```python
from build123d import *

# Parameters (mm, degrees)
F0_W     = 145
F0_H     = 580
F1_DEPTH = 10
F2_W     = 125
F2_H     = 560
F3_DEPTH = 10
F4_R     = 1


with BuildPart() as f1:
    # F0 (on Top) → F1 (new body)
    with BuildSketch(Plane.XY):
        with Locations((-112.119565, 4.486432)):
            Rectangle(F0_W, F0_H)
    extrude(amount=F1_DEPTH)

    # F2 (on face) → F3 (join)
    with BuildSketch(Plane(origin=(0, 0, 0), x_dir=(1, 0, 0), z_dir=(0, 0, -1))):
        with Locations((-112.119565, -4.486432)):
            Rectangle(F2_W, F2_H)
    extrude(amount=F3_DEPTH)

    # F4
    f4_edges = [f1.edges().sort_by_distance(p)[0] for p in [
        (-49.619565, 4.486432, -10),
        (-112.119565, -275.513568, -10),
        (-174.619565, 4.486432, -10),
        (-112.119565, 284.486432, -10),
        (-184.619565, 4.486432, 0),
        (-49.619565, -275.513568, -5),
        (-174.619565, -275.513568, -5),
        (-112.119565, -275.513568, 0),
        (-49.619565, 284.486432, -5),
        (-49.619565, 4.486432, 0),
        (-39.619565, -285.513568, 5),
        (-39.619565, 294.486432, 5),
        (-39.619565, 4.486432, 0),
        (-39.619565, 4.486432, 10),
        (-184.619565, -285.513568, 5),
        (-112.119565, -285.513568, 0),
        (-112.119565, -285.513568, 10),
        (-184.619565, 294.486432, 5),
        (-184.619565, 4.486432, 10),
        (-112.119565, 294.486432, 0),
        (-112.119565, 294.486432, 10),
        (-174.619565, 284.486432, -5),
        (-112.119565, 284.486432, 0),
        (-174.619565, 4.486432, 0),
    ]]
    fillet(f4_edges, radius=F4_R)


solid = f1.part
```
Geometry check sheet. Reference: the model listing, model coordinates, mm. Coordinates: 2 decimals unless noted, no trailing zeros. Loops run counter-clockwise (first coordinate to the right, second up) from the corner with the lowest first, then second, coordinate; pieces in that order, holes last.
Item 1: Sectioned sample at C-C, the plane x = -141. Record the boundary of the cut face in (y, z).
Item 2: Sectioned sample at A-A, the plane y = -56.5. Record the boundary of the cut face in (x, z), then the cut area to 3 significant figures.
Item 3: Go/stop test with flat-tipped pins: pin 1 Ø2.5 at (x, z) = (-114, -4) entering from +Y; pin 2 Ø2 at (y, z) = (-95.5, -2) entering from -X; pin 3 Ø4 at (x, z) = (-140.5, -4.5) entering from -Y. Record where each tip stops, or that it passes through.
Item 4: Thickness scan on line 1 (X direction, y = -126, z = 9.25); line 2 (X direction, y = -84, z = -7); line 3 (Y direction, x = -56, z = -4). Record the ranges inside material, lowest first.
Item 5: Sectioned sample at B-B, the plane z = -6. Record the boundary of the cut face in (x, y), then the cut area to 3 significant figures.
Check result:
1. outline: (-285.51, 1) arc R1 ccw to (-284.51, 0) - (-276.51, 0) arc R1 cw to (-275.51, -1) - (-275.51, -9) arc R1 ccw to (-274.51, -10) - (283.49, -10) arc R1 ccw to (284.49, -9) - (284.49, -1) arc R1 cw to (285.49, 0) - (293.49, 0) arc R1 ccw to (294.49, 1) - (294.49, 9) arc R1 ccw to (293.49, 10) - (-284.51, 10) arc R1 ccw to (-285.51, 9) - close
2. outline: (-184.62, 1) arc R1 ccw to (-183.62, 0) - (-175.62, 0) arc R1 cw to (-174.62, -1) - (-174.62, -9) arc R1 ccw to (-173.62, -10) - (-50.62, -10) arc R1 ccw to (-49.62, -9) - (-49.62, -1) arc R1 cw to (-48.62, 0) - (-40.62, 0) arc R1 ccw to (-39.62, 1) - (-39.62, 9) arc R1 ccw to (-40.62, 10) - (-183.62, 10) arc R1 ccw to (-184.62, 9) - close
2. area: 2,700 mm2
3. pin 1: stops at y = 284.49
3. pin 2: stops at x = -174.62
3. pin 3: stops at y = -275.51
4. line 1: x = -184.59 to -39.65
4. line 2: x = -174.62 to -49.62
4. line 3: y = -275.51 to 284.49
5. outline: (-174.62, -274.51) arc R1 ccw to (-173.62, -275.51) - (-50.62, -275.51) arc R1 ccw to (-49.62, -274.51) - (-49.62, 283.49) arc R1 ccw to (-50.62, 284.49) - (-173.62, 284.49) arc R1 ccw to (-174.62, 283.49) - close
5. area: 70,000 mm2
